Geometry: final body of the model. Coordinates: model frame, mm. Face numbers are marked on the shaded views. A direction names the side the tool comes from. Give positions to 0.01 mm unless a question says otherwise; leave off trailing zeros. Loops run counter-clockwise (first coordinate to the right, second up) from the corner with the lowest first, then second, coordinate; pieces in that order, holes last.
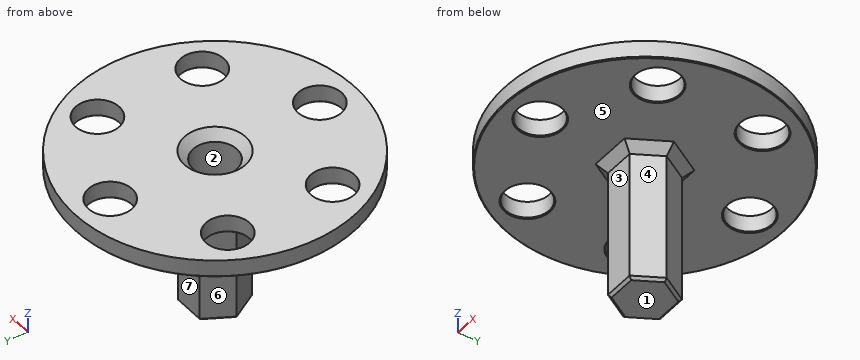
from build123d import *

# Parameters (mm, degrees)
SKETCH1_R           = 32
BOSS_EXTRUDE1_DEPTH = 4
SKETCH2_R           = 5
CUT_EXTRUDE1_DEPTH  = 46.431266766
CIRPATTERN1_COUNT   = 6
BOSS_EXTRUDE2_DEPTH = 32
CHAMFER1_SIZE       = 2
CHAMFER2_SIZE       = 0.2
SKETCH4_R           = 5
CUT_EXTRUDE2_DEPTH  = 32
CHAMFER3_SIZE       = 0.6
CHAMFER4_SIZE       = 5
CHAMFER5_SIZE       = 2
SCALE1_SCALE        = 0.4


with BuildPart() as part:
    # Sketch1 → Boss-Extrude1 (new body)
    with BuildSketch(Plane.XY):
        Circle(SKETCH1_R)
    extrude(amount=-BOSS_EXTRUDE1_DEPTH)

    # Sketch2 → Cut-Extrude1 (cut, through all)
    with BuildSketch(Plane.XY):
        with Locations((0, 24)):
            Circle(SKETCH2_R)
    cut_extrude1 = extrude(amount=-CUT_EXTRUDE1_DEPTH, mode=Mode.SUBTRACT)

    # CirPattern1: Cut-Extrude1 ×6 about axis
    cirpattern1_axis = Axis((0, 0, 0), (0, 0, 1))
    for i in range(1, CIRPATTERN1_COUNT):
        add(cut_extrude1.rotate(cirpattern1_axis, i * 360 / CIRPATTERN1_COUNT), mode=Mode.SUBTRACT)

    # Sketch3 → Boss-Extrude2 (add)
    with BuildSketch(Plane(origin=(0, 0, -4), x_dir=(-1, 0, 0), z_dir=(0, 0, -1))):
        Polygon((-3.464101615, 6), (-6.92820323, 0), (-3.464101615, -6), (3.464101615, -6), (6.92820323, 0), (3.464101615, 6), align=None)
    extrude(amount=BOSS_EXTRUDE2_DEPTH)

    # Chamfer1
    chamfer1_edges = [part.edges().sort_by_distance(p)[0] for p in [
        (0, 6, -4),
        (5.196152423, 3, -4),
        (5.196152423, -3, -4),
        (0, -6, -4),
        (-5.196152423, -3, -4),
        (-5.196152423, 3, -4),
    ]]
    chamfer(chamfer1_edges, length=CHAMFER1_SIZE)

    # Chamfer2
    chamfer2_edges = [part.edges().sort_by_distance(p)[0] for p in [
        (-23.284609691, 7.669872981, -4),
        (-18.284609691, -16.330127019, -4),
        (5, -24, -4),
        (23.284609691, -7.669872981, -4),
        (18.284609691, 16.330127019, -4),
        (-32, 0, -4),
        (-5, 24, -4),
    ]]
    chamfer(chamfer2_edges, length=CHAMFER2_SIZE)

    # Sketch4 → Cut-Extrude2 (cut)
    with BuildSketch(Plane.XY):
        Circle(SKETCH4_R)
    extrude(amount=-CUT_EXTRUDE2_DEPTH, mode=Mode.SUBTRACT)

    # Chamfer3
    chamfer3_edges = [part.edges().sort_by_distance(p)[0] for p in [
        (0, 6, -36),
        (5.196152423, 3, -36),
        (5.196152423, -3, -36),
        (0, -6, -36),
        (-5.196152423, -3, -36),
        (-5.196152423, 3, -36),
    ]]
    chamfer(chamfer3_edges, length=CHAMFER3_SIZE)

    # Chamfer4
    chamfer4_edges = [part.edges().sort_by_distance(p)[0] for p in [
        (-5, 0, -32),
    ]]
    chamfer(chamfer4_edges, length=CHAMFER4_SIZE)

    # Chamfer5
    chamfer5_edges = [part.edges().sort_by_distance(p)[0] for p in [
        (-5, 0, 0),
    ]]
    chamfer(chamfer5_edges, length=CHAMFER5_SIZE)


with BuildPart() as part_1:
    # Scale1: scaled about (0, 0, -5.463972753)
    add(part.part.scale(SCALE1_SCALE).moved(Location((0, 0, -3.278383652))))


solid = part_1.part
Item 1: Draft query along Y for the marked faces 1, 2 and 3. Return one class per face: +Y half, -Y half, draft (parallel to the pull), parting line (faces both ways), or undercut.
Values follow:
face 1: draft
face 2: undercut
face 3: -Y half
Item 2: Pin query (flat end, axial travel): pin 1 (2.5 mm diameter, centred on x = -8.31, y = -4.8, fed in from +Z); pin 2 (5 mm diameter, centred on x = 8.31, y = -4.8, fed in from -Z); pin 3 (4.5 mm diameter, centred on x = 0, y = -9.6, fed in from +Z); pin 4 (0.8 mm diameter, centred on x = -0.5, z = -10, fed in from +Y). Return the tip coordinate at first contact, or that it passes through.
Values follow:
pin 1: passes through
pin 2: stops at z = -4.88
pin 3: stops at z = -3.28
pin 4: stops at y = 2.4
Item 3: Set-up query: the marked faces 4, 5, 6 and 7. Return all of +Z, -Z, +X, -X, +Y, -Y with unobstructed straight access to the full face (end or side cutting, diameter ignored); none if empty.
Values follow:
face 4: -Z, +X, -Y
face 5: -Z
face 6: -Z, -X, +Y
face 7: -Z, +X, -X, +Y
Item 4: Ray query, probe 1 along Z at (x, y) = (7, -3); probe 2 along Y at (x, z) = (0, -4.05); probe 3 along X at (y, z) = (-0.75, -14.5). Return the intervals inside material, ascending.
Values follow:
probe 1: z = -4.88 to -3.28
probe 2: y = -12.8 to -11.6, -7.6 to -2.03, 2.03 to 7.6, 11.6 to 12.8
probe 3: x = -2.34 to -1.39, 1.39 to 2.34
Item 5: Section query B-B on y = -3.75. Give the number of separate pieces and of enclosed holes in the cut face, plus the area to 3 significant figures.
Values follow:
separate pieces: 3
enclosed holes: 0
area: 28.2 mm2
Item 6: Section query A-A on z = -6. Return loops of the section in (x, y), plus the area to 3 significant figures.
Values follow:
outline: (-2.77, 0) - (-1.39, -2.4) - (1.39, -2.4) - (2.77, 0) - (1.39, 2.4) - (-1.39, 2.4) - close; hole circle Ø4 at (0, 0)
area: 7.39 mm2
